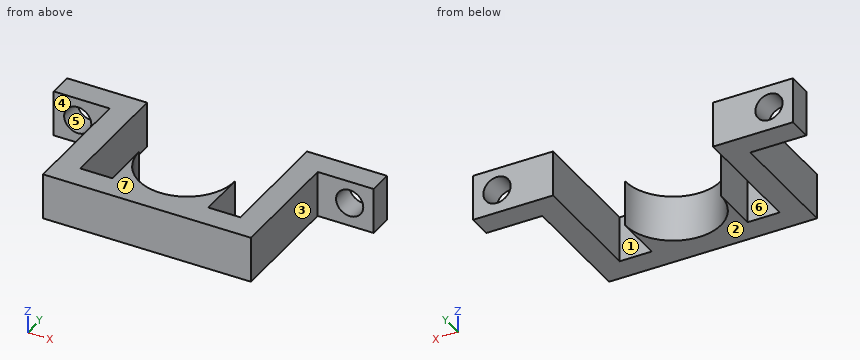
```python
from build123d import *

# Parameters (mm, degrees)
PAD032_DEPTH  = 5.75
SKETCH096_W   = 3
SKETCH096_H   = 5.75
PAD033_DEPTH  = 18
SKETCH097_W   = 7
SKETCH097_H   = 3
PAD034_DEPTH  = 5.75
SKETCH098_R   = 1.7
HOLE019_DEPTH = 25


with BuildPart() as part:
    # Sketch095 → Pad032 (new body)
    with BuildSketch(Plane.XY):
        with BuildLine():
            Line((-10, 0), (-10, -3))
            Line((-10, -3), (10, -3))
            Line((10, -3), (10, 0))
            Line((10, 0), (6, 0))
            Line((6, 6), (6, 0))
            ThreePointArc((-6, 6), (0, 0), (6, 6))
            Line((-6, 0), (-6, 6))
            Line((-6, 0), (-10, 0))
        make_face()
    extrude(amount=PAD032_DEPTH)

    # Sketch096 → Pad033 (join)
    with BuildSketch(Plane.XZ.offset(3)):
        with Locations((-11.5, 2.875)):
            Rectangle(SKETCH096_W, SKETCH096_H)
        with Locations((11.5, 2.875)):
            Rectangle(SKETCH096_W, SKETCH096_H)
    extrude(amount=-PAD033_DEPTH)

    # Sketch097 (on Face7 of Pad033) → Pad034 (join)
    with BuildSketch(Plane.XY.offset(5.75)):
        with Locations((-16.5, 13.5)):
            Rectangle(SKETCH097_W, SKETCH097_H)
        with Locations((16.5, 13.5)):
            Rectangle(SKETCH097_W, SKETCH097_H)
    extrude(amount=-PAD034_DEPTH)

    # Sketch098 (on Face26 of Pad034) → Hole019 (cut)
    with BuildSketch(Plane.XZ.offset(-12)):
        with Locations((-17, 2.95)):
            Circle(SKETCH098_R)
        with Locations((17, 2.95)):
            Circle(SKETCH098_R)
    extrude(amount=-HOLE019_DEPTH, mode=Mode.SUBTRACT)


with BuildPart() as part_1:
    # Body014 placement: moved
    add(part.part.moved(Location((0, 114, 205.555))))


solid = part_1.part
```
Check sheet for the modelled part. Datum: model origin and axes. Units: mm. Face numbers are marked on the shaded views. A direction names the side the tool comes from. Round coordinates to 2 decimals unless told otherwise and drop trailing zeros. Order: outer loops, then holes, each group sorted by start corner. A loop starts at its lowest first (then second) coordinate and runs counter-clockwise, first axis right, second up. Notation, with made-up numbers: (79, 16) - (136, 16) arc R19 ccw to (136, 32) - close; hole circle Ø4 at (80, -33). An arc over 180 degrees is marked (long way). Write item = value, one per line.
Q1. Go/stop test with flat-tipped pins: pin 1 (1.7 mm diameter, centred on x = -17.5, z = 207, fed in from -Y); pin 2 (1 mm diameter, centred on x = 2.5, z = 209, fed in from +Y); pin 3 (1.7 mm diameter, centred on y = 117, z = 209.5, fed in from -X). Record where each tip stops, or that it passes through.
Computed:
pin_1 = 126
pin_2 = 114.8
pin_3 = -13
Q2. Section check D-D (z = 206.35). Record the boundary of the cut face in (x, y), and give its area (3 significant figures).
Computed:
outline = (-20, 126) - (-13, 126) - (-13, 111) - (13, 111) - (13, 126) - (20, 126) - (20, 129) - (10, 129) - (10, 114) - (6, 114) - (6, 120) arc R6 cw to (-6, 120) - (-6, 114) - (-10, 114) - (-10, 129) - (-20, 129) - close
area = 225 mm^2
Q3. Section check C-C (y = 127.5). Record the boundary of the cut face in (x, z) (3 decimals).
Computed:
outline = (-20, 205.555) - (-10, 205.555) - (-10, 211.305) - (-20, 211.305) - close; (10, 205.555) - (20, 205.555) - (20, 211.305) - (10, 211.305) - close; hole circle Ø3.4 at (-17, 208.505); hole circle Ø3.4 at (17, 208.505)
Q4. Tool access check on the marked faces 1, 2, 3 and 4. Record the directions out of +Z, -Z, +X, -X, +Y, -Y that give a thin tool (end or side, any length) a straight path to the whole face; none if there is none.
Computed:
face_1 = +Z, -Z, +Y
face_2 = -Z, +X, -X, +Y, -Y
face_3 = +Z, -Z, +X, -Y
face_4 = +Z, -Z, -X, -Y
Q5. Section check A-A (y = 123.5). Record the boundary of the cut face in (x, z) (3 decimals).
Computed:
outline = (-13, 205.555) - (-10, 205.555) - (-10, 211.305) - (-13, 211.305) - close; (10, 205.555) - (13, 205.555) - (13, 211.305) - (10, 211.305) - close
Q6. Draft check along Z on the marked faces 5, 6 and 7. Enter one of: pulls with the +Z half, pulls with the -Z half, needs draft (parallel to the pull), parting line crosses it, or undercut.
Computed:
face_5 = undercut
face_6 = needs draft
face_7 = pulls with the +Z half
Q7. Section check B-B (x = 17). Record the boundary of the cut face in (y, z) (3 decimals).
Computed:
outline = (126, 205.555) - (129, 205.555) - (129, 206.805) - (126, 206.805) - close; (126, 210.205) - (129, 210.205) - (129, 211.305) - (126, 211.305) - close
Q8. Thickness scan on line 1 along Z through (x, y) = (17, 127.9) (3 decimals); line 2 along X through (y, z) = (123.5, 207.7); line 3 along X through (y, z) = (117.25, 206.3). Record the ranges inside material, lowest first.
Computed:
line_1 = 205.555 to 206.805, 210.205 to 211.305
line_2 = -13 to -10, 10 to 13
line_3 = -13 to -10, -6 to -5.33, 5.33 to 6, 10 to 13
